```python
from build123d import *

# Parameters (mm, degrees)
SKETCH1_R           = 3.175
SKETCH1_R_2         = 11
BOSS_EXTRUDE1_DEPTH = 10
FILLET3_R           = 2


with BuildPart() as part:
    # Sketch1 → Boss-Extrude1 (new body)
    with BuildSketch(Plane.XY):
        with BuildLine():
            Line((-44.45, -12.7), (-44.45, 12.7))
            Line((-44.45, 12.7), (36.468145579, 12.7))
            ThreePointArc((36.468145579, 12.7), (39.105886278, 14.015721477), (41.95, 14.790199458))
            Line((41.95, 14.790199458), (46.95, 14.790199458))
            ThreePointArc((46.95, 14.790199458), (59.45, 0), (46.95, -14.790199458))
            Line((46.95, -14.790199458), (41.95, -14.790199458))
            ThreePointArc((41.95, -14.790199458), (39.105886278, -14.015721477), (36.468145579, -12.7))
            Line((36.468145579, -12.7), (-44.45, -12.7))
        make_face()
        with Locations((-31.75, 0)):
            Circle(SKETCH1_R, mode=Mode.SUBTRACT)
        with Locations((44.45, 0)):
            Circle(SKETCH1_R_2, mode=Mode.SUBTRACT)
        with Locations((-6.35, 0)):
            Circle(SKETCH1_R, mode=Mode.SUBTRACT)
    extrude(amount=BOSS_EXTRUDE1_DEPTH)

    # Fillet3
    fillet3_edges = [part.edges().sort_by_distance(p)[0] for p in [
        (-44.45, -12.7, 5),
        (-44.45, 12.7, 5),
    ]]
    fillet(fillet3_edges, radius=FILLET3_R)


solid = part.part
```
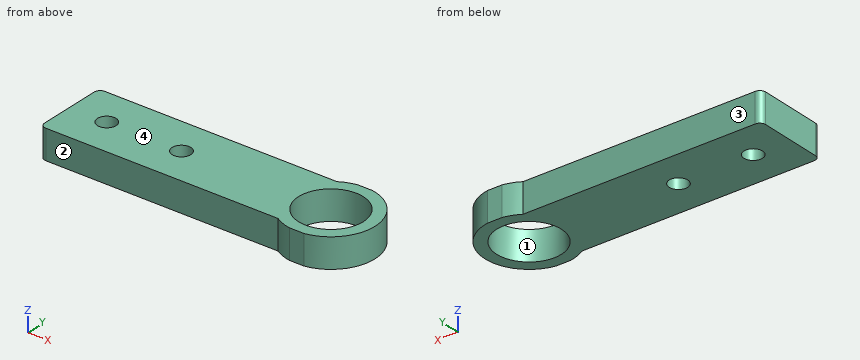
Source: CAD feature listing. Evaluate the final solid. Frame: model axes, mm. Face numbers are marked on the shaded views. Give positions to 0.01 mm unless a question says otherwise; leave off trailing zeros. Loops run counter-clockwise (first coordinate to the right, second up) from the corner with the lowest first, then second, coordinate; pieces in that order, holes last. Notation, with made-up numbers: (42, 26.5) -> (92, 26.5) arc R23 ccw to (92, 64.5) -> close; hole circle Ø11 at (-40, 3). An arc over 180 degrees is marked (long way). Use a Markdown table: item, result. Add a question column.
(1) Section query D-D (y = -6.75). Output: boundary loops of the cut face in (x, z), then the cut area to 3 significant figures.
(2) Section query B-B (z = 4.75). Output: boundary loops of the cut face in (x, y) (3 decimals).
(3) Pull-direction query (Y, two-part tool) for the marked faces 1, 2, 3 and 4; classes: +Y half, -Y half, draft (parallel to the pull), parting line (faces both ways), or undercut.
(4) Section query A-A (x = 44.45). Output: boundary loops of the cut face in (y, z).
(5) Section query C-C (y = 0). Output: boundary loops of the cut face in (x, z) (3 decimals), then the cut area to 3 significant figures.
(6) Ray query, line 1 (Y direction, x = -31.75, z = 2.75) (3 decimals); line 2 (Y direction, x = 44.5, z = 1); line 3 (Y direction, x = 7.5, z = 5). Return the intervals inside material, ascending.
(7) First-contact query: pin 1 Ø1.5 at (x, z) = (-4.5, 6.5) entering from -Y; pin 2 Ø3 at (x, z) = (-11.5, 5) entering from +Y. Flat tips, straight axial feed; report the tip coordinate or a pass-through.
Checked values:
| question | item | result |
|---|---|---|
| 1 | outline | (-44.45, 0) -> (35.76, 0) -> (35.76, 10) -> (-44.45, 10) -> close; (53.14, 0) -> (57.85, 0) -> (57.85, 10) -> (53.14, 10) -> close |
| 1 | area | 849 mm^2 |
| 2 | outline | (-44.45, -10.7) arc R2 ccw to (-42.45, -12.7) -> (36.468, -12.7) arc R15 ccw to (41.95, -14.79) -> (46.95, -14.79) arc R15 ccw to (46.95, 14.79) -> (41.95, 14.79) arc R15 ccw to (36.468, 12.7) -> (-42.45, 12.7) arc R2 ccw to (-44.45, 10.7) -> close; hole circle Ø6.35 at (-31.75, 0); hole circle Ø6.35 at (-6.35, 0); hole circle Ø22 at (44.45, 0) |
| 3 | face 1 | undercut |
| 3 | face 2 | -Y half |
| 3 | face 3 | +Y half |
| 3 | face 4 | draft |
| 4 | outline | (-14.79, 0) -> (-11, 0) -> (-11, 10) -> (-14.79, 10) -> close; (11, 0) -> (14.79, 0) -> (14.79, 10) -> (11, 10) -> close |
| 5 | outline | (-44.45, 0) -> (-34.925, 0) -> (-34.925, 10) -> (-44.45, 10) -> close; (-28.575, 0) -> (-9.525, 0) -> (-9.525, 10) -> (-28.575, 10) -> close; (-3.175, 0) -> (33.45, 0) -> (33.45, 10) -> (-3.175, 10) -> close; (55.45, 0) -> (59.45, 0) -> (59.45, 10) -> (55.45, 10) -> close |
| 5 | area | 692 mm^2 |
| 6 | line 1 | -12.7 to -3.175, 3.175 to 12.7 |
| 6 | line 2 | -14.79 to -11, 11 to 14.79 |
| 6 | line 3 | -12.7 to 12.7 |
| 7 | pin 1 | y = -12.7 |
| 7 | pin 2 | y = 12.7 |
